Can you work these out from the drawing? Everything is in mm from the part's minimum corner. Round coordinates to 2 decimals unless told otherwise and drop trailing zeros. Loops run counter-clockwise (first coordinate to the right, second up) from the corner with the lowest first, then second, coordinate; pieces in that order, holes last. Notation, with made-up numbers: (6.5, 23.5) - (47.5, 23.5) arc R22 cw to (47.5, 52.5) - close; hole circle Ø5 at (-10, 21.25). An arc over 180 degrees is marked (long way). Put each result on its own line as item: value. Start each with the question number.
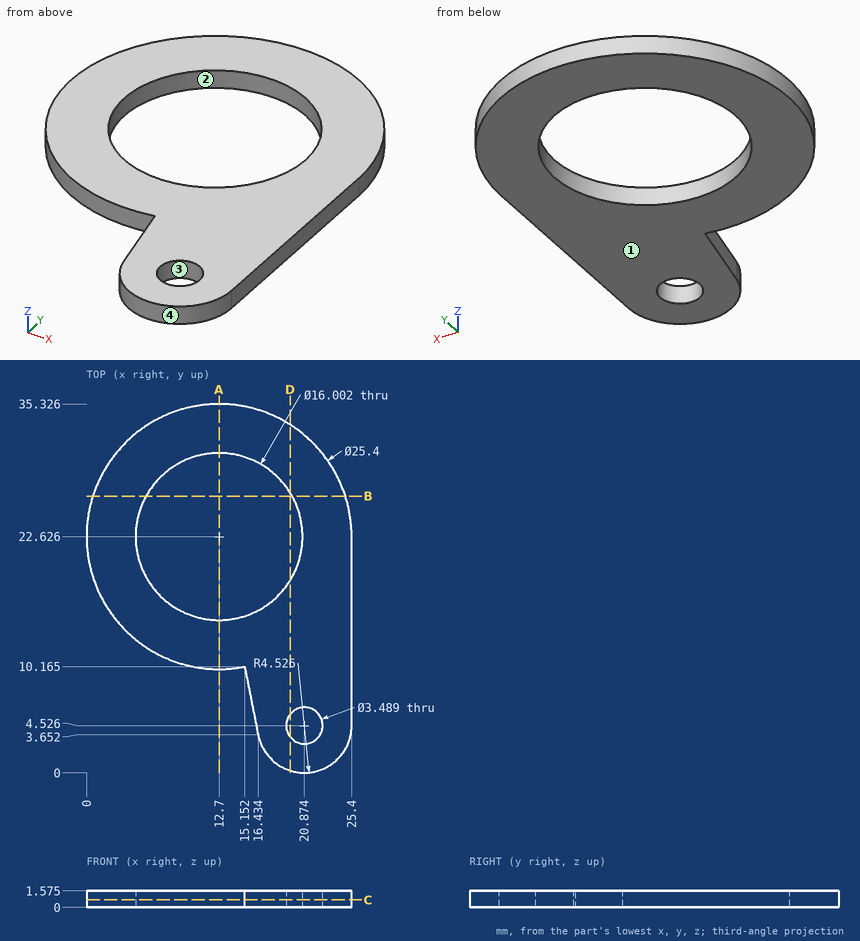
Item 1: Suppose I cut it at C-C, the plane z = 0.7. List the corners of the cut face in (x, y) for me (1 decimal).
Item 2: Suppose I cut it at B-B, the plane y = 26.5. List the corners of the cut face in (x, z) for me (1 decimal).
Item 3: Thinking about a two-plate mould opening in X: for the marked faces 1, 2, 3 and 4, which applies, released by +X, released by -X, zero draft, split by the parting line, or undercut?
Item 4: I need wall thicknesses on line 1 (Y direction, x = 12.7, z = 0.55) (1 decimal); line 2 (X direction, y = 22.5, z = 0.9); line 3 (X direction, y = 4, z = 1.1) (1 decimal). Which ranges of each line are inside material? Lowest first, please. Write a range as from..to.
Item 5: Suppose I cut it at A-A, the plane x = 12.7. List the corners of the cut face in (y, z) for me (1 decimal).
Item 6: Will this pin go through, and if not, where does the flat tip stop? P1, Ø8, axis at x = 16.5, y = 25.5, coming from the +Z side (1 decimal).
Item 7: Suppose I cut it at D-D, the plane x = 19.5. List the corners of the cut face in (y, z) for me (1 decimal).
Numbers:
1. outline: (15.2, 10.2) - (16.4, 3.7) arc R4.5 ccw to (25.4, 4.5) - (25.4, 22.6) arc R12.7 ccw (long way) to start; hole circle Ø16 at (12.7, 22.6); hole circle Ø3.5 at (20.9, 4.5)
2. outline: (0.6, 0) - (5.7, 0) - (5.7, 1.6) - (0.6, 1.6) - close; (19.7, 0) - (24.8, 0) - (24.8, 1.6) - (19.7, 1.6) - close
3. face 1: zero draft
3. face 2: undercut
3. face 3: undercut
3. face 4: split by the parting line
4. line 1: 9.9..14.6, 30.6..35.3
4. line 2: 0..4.7, 20.7..25.4
4. line 3: 16.4..19.2, 22.5..25.4
5. outline: (9.9, 0) - (14.6, 0) - (14.6, 1.6) - (9.9, 1.6) - close; (30.6, 0) - (35.3, 0) - (35.3, 1.6) - (30.6, 1.6) - close
6. P1: z = 1.6
7. outline: (0.2, 0) - (3.5, 0) - (3.5, 1.6) - (0.2, 1.6) - close; (5.6, 0) - (18.4, 0) - (18.4, 1.6) - (5.6, 1.6) - close; (26.8, 0) - (33.4, 0) - (33.4, 1.6) - (26.8, 1.6) - close
